Study the drawing (mm; zero at the part's minimum x, y, z) and answer. Give positions to 0.01 mm unless a question says otherwise; leave off trailing zeros. Loops run counter-clockwise (first coordinate to the right, second up) from the corner with the lowest first, then second, coordinate; pieces in that order, holes last. Notation, with made-up numbers: (12.25, -1) - (61.25, -1) arc R18 cw to (61.25, 22) - close; hole circle Ø2 at (-6, 85.25). An arc over 180 degrees is marked (long way). Write item = value, one per line. Start each with the question number.
1) The part is cut by section B-B on y = 25. Write down the section's boundary in (x, z), plus the area to 3 significant figures.
2) Flat-ended cylindrical pins translate along their axes: P1, Ø4, axis at y = 9, z = 34, coming from the +X side; P2, Ø10, axis at y = 14, z = 6.5, coming from the +X side (1 decimal); P3, Ø6, axis at x = 41.5, y = 19, coming from the +Z side. Find the tip coordinate at first contact, or state that the pin passes through.
3) Consider probe 1 along Z at (x, y) = (23.5, 8.5); probe 2 along X at (y, z) = (29, 7) (1 decimal); probe 3 along Z at (x, y) = (32.5, 12) (1 decimal). Determine where each line is inside the solid, lowest interval first.
4) The part is cut by section A-A on y = 35. Write down the section's boundary in (x, z), plus the area to 3 significant figures.
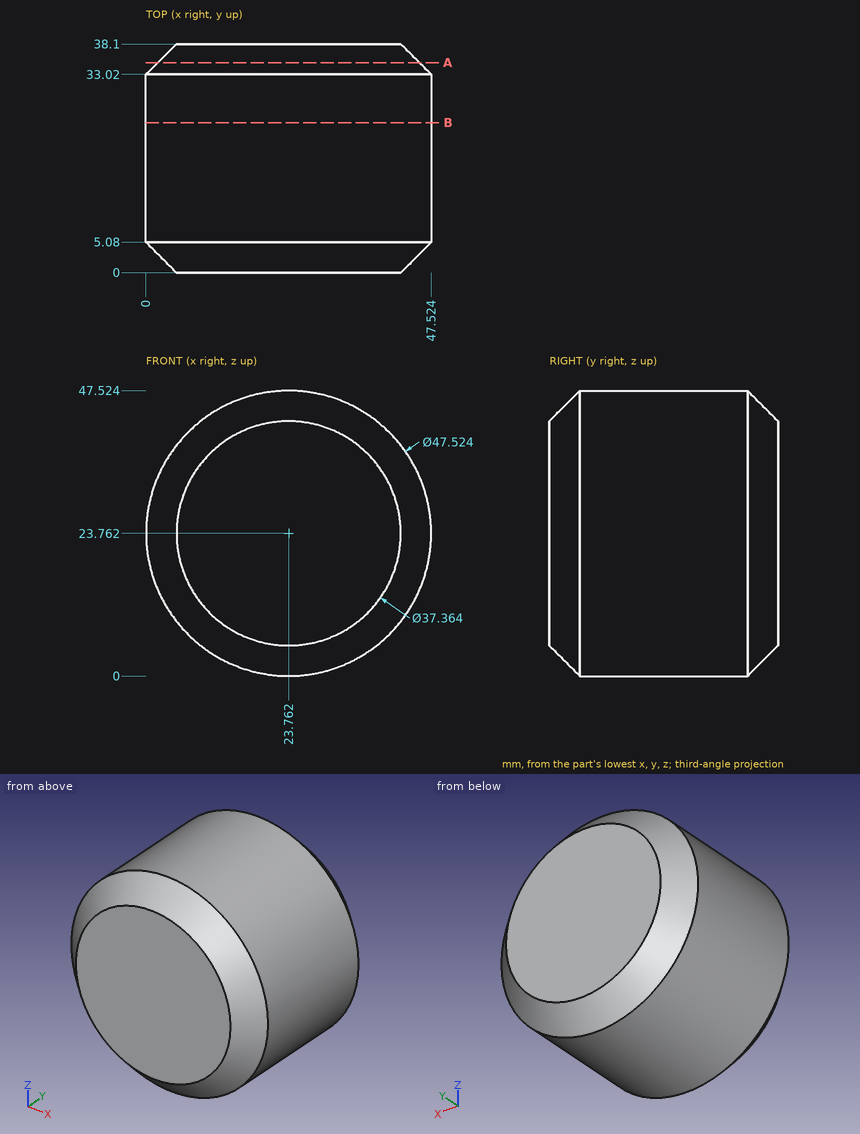
Answer below:
q1.outline = circle Ø47.52 at (23.76, 23.76)
q1.area = 1,770 mm2
q2.P1 = 46.05
q2.P2 = 44.1
q2.P3 = 42.4
q3.probe_1 = 0 to 47.52
q3.probe_2 = 6.9 to 40.6
q3.probe_3 = 1.7 to 45.9
q4.outline = circle Ø43.56 at (23.76, 23.76)
q4.area = 1,490 mm2
